Could you check a few things on this model? Use its own coordinates, in mm. Face numbers are marked on the shaded views. A direction names the side the tool comes from. Round coordinates to 2 decimals unless told otherwise and drop trailing zeros. Write each loop counter-clockwise with the first axis right and the second up, starting at its lowest first coordinate (ties: lowest second). Pieces come first, ordered by that corner, then holes. Notation, with made-up numbers: (52.25, 0.25) -> (67.25, 0.25) arc R33 cw to (67.25, 30.25) -> close; hole circle Ø8 at (71, -1.75). An arc over 180 degrees is marked (long way). Answer in a Markdown table with one row per item.
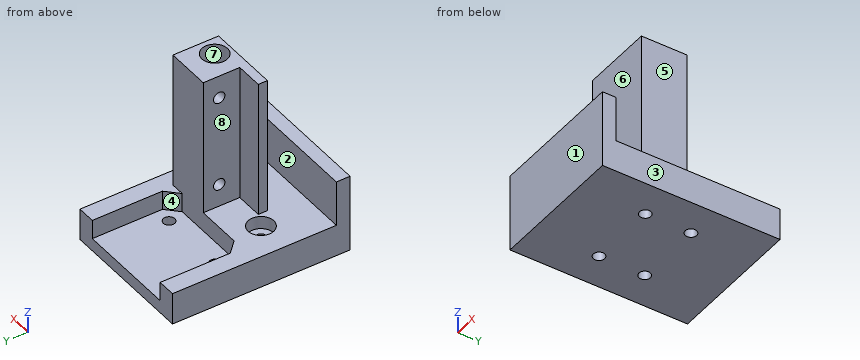
from build123d import *

# Parameters (mm, degrees)
SKETCH016_W     = 30
SKETCH016_H     = 38.9
SKETCH016_R     = 1.25
PAD010_DEPTH    = 7
POCKET005_DEPTH = 4.2
SKETCH020_R     = 2.8
POCKET006_DEPTH = 2.8
SKETCH021_R     = 2.8
PAD011_DEPTH    = 30
SKETCH022_R     = 1.25
POCKET007_DEPTH = 5.3
SKETCH026_W     = 30
SKETCH026_H     = 3
PAD015_DEPTH    = 10


with BuildPart() as part:
    # Sketch016 (on Face1 of ReferencePad007) → Pad010 (new body)
    with BuildSketch(Plane.XY.offset(3.5)):
        with Locations((0, 132.225)):
            Rectangle(SKETCH016_W, SKETCH016_H)
        with Locations((-7.5, 137.225)):
            Circle(SKETCH016_R, mode=Mode.SUBTRACT)
        with Locations((-7.5, 127.225)):
            Circle(SKETCH016_R, mode=Mode.SUBTRACT)
        with Locations((7.5, 137.225)):
            Circle(SKETCH016_R, mode=Mode.SUBTRACT)
        with Locations((7.5, 127.225)):
            Circle(SKETCH016_R, mode=Mode.SUBTRACT)
    extrude(amount=PAD010_DEPTH)

    # Sketch019 (on Face10 of Pad010) → Pocket005 (cut)
    with BuildSketch(Plane.XY.offset(10.5)):
        Polygon((-8.411624, 133.725), (-11, 136.313376), (-11, 151.675), (11, 151.675), (11, 136.313376), (8.411624, 133.725), align=None)
    extrude(amount=-POCKET005_DEPTH, mode=Mode.SUBTRACT)

    # Sketch020 (on Face5 of Pocket005) → Pocket006 (cut)
    with BuildSketch(Plane.XY.offset(10.5)):
        with Locations((-7.5, 127.225)):
            Circle(SKETCH020_R)
        with Locations((7.5, 127.225)):
            Circle(SKETCH020_R)
    extrude(amount=-POCKET006_DEPTH, mode=Mode.SUBTRACT)

    # Sketch021 (on Face5 of Pocket006) → Pad011 (join)
    with BuildSketch(Plane.XY.offset(10.5)):
        Polygon((-4.411624, 123.725), (11.411624, 123.725), (11.411624, 133.725), (1.588376, 133.725), (1.588376, 125.725), (-4.411624, 125.725), align=None)
        with Locations((7.5, 127.225)):
            Circle(SKETCH021_R, mode=Mode.SUBTRACT)
    extrude(amount=PAD011_DEPTH)

    # Sketch022 (on Face14 of Pad011) → Pocket007 (cut)
    with BuildSketch(Plane(origin=(1.588376, 0, 8), x_dir=(0, -1, 0), z_dir=(-1, 0, 0))):
        with Locations((-130.225, 27.5)):
            Circle(SKETCH022_R)
        with Locations((-130.225, 7.5)):
            Circle(SKETCH022_R)
    extrude(amount=-POCKET007_DEPTH, mode=Mode.SUBTRACT)

    # Sketch026 (on Face5 of Pocket007) → Pad015 (join)
    with BuildSketch(Plane.XY.offset(10.5)):
        with Locations((0, 114.275)):
            Rectangle(SKETCH026_W, SKETCH026_H)
    extrude(amount=PAD015_DEPTH)


solid = part.part
1) Thinking about a two-plate mould opening in Y: for the marked faces 1, 2 and 3, which applies, +Y half, -Y half, draft (parallel to the pull), parting line (faces both ways), or undercut?
Findings:
| item | result |
|---|---|
| face 1 | -Y half |
| face 2 | undercut |
| face 3 | draft |
2) Please list where these lines run through material, in increasing order: line 1 (Y direction, x = 7.5, z = 5.65) (3 decimals); line 2 (Y direction, x = 7.5, z = 26) (3 decimals); line 3 (Y direction, x = 3.9, z = 35.5) (3 decimals).
Findings:
| item | result |
|---|---|
| line 1 | y = 112.775 to 125.975, 128.475 to 135.975, 138.475 to 151.675 |
| line 2 | y = 123.725 to 124.425, 130.025 to 133.725 |
| line 3 | y = 123.725 to 128.975, 131.475 to 133.725 |
3) Imagine slicing it at B-B, the plane z = 12. Please give me the cut outline in (x, y) (3 decimals).
Findings:
| item | result |
|---|---|
| outline | (-15, 112.775) -> (15, 112.775) -> (15, 115.775) -> (-15, 115.775) -> close; (-4.412, 123.725) -> (11.412, 123.725) -> (11.412, 133.725) -> (1.588, 133.725) -> (1.588, 125.725) -> (-4.412, 125.725) -> close; hole circle Ø5.6 at (7.5, 127.225) |
4) For the marked faces 4, 5, 6, 7 and 8, which set-ups out of +Z, -Z, +X, -X, +Y, -Y let a thin tool reach every point of the face, with its end or its side?
Findings:
| item | result |
|---|---|
| face 4 | +Z, +Y |
| face 5 | +Z, +X, +Y |
| face 6 | +Z, +X, -X |
| face 7 | +Z |
| face 8 | +Z, -X, +Y |
5) Imagine slicing it at A-A, the plane x = 7.5. Please give me the cut outline in (y, z) (3 decimals), plus the area to 3 significant figures.
Findings:
| item | result |
|---|---|
| outline | (112.775, 3.5) -> (125.975, 3.5) -> (125.975, 7.7) -> (124.425, 7.7) -> (124.425, 40.5) -> (123.725, 40.5) -> (123.725, 10.5) -> (115.775, 10.5) -> (115.775, 20.5) -> (112.775, 20.5) -> close; (128.475, 3.5) -> (135.975, 3.5) -> (135.975, 6.3) -> (133.725, 6.3) -> (133.725, 40.5) -> (130.025, 40.5) -> (130.025, 7.7) -> (128.475, 7.7) -> close; (138.475, 3.5) -> (151.675, 3.5) -> (151.675, 6.3) -> (138.475, 6.3) -> close |
| area | 326 mm^2 |
6) Imagine slicing it at C-C, the plane x = -0.5. Please give me the cut outline in (y, z) (3 decimals).
Findings:
| item | result |
|---|---|
| outline | (112.775, 3.5) -> (151.675, 3.5) -> (151.675, 6.3) -> (133.725, 6.3) -> (133.725, 10.5) -> (125.725, 10.5) -> (125.725, 40.5) -> (123.725, 40.5) -> (123.725, 10.5) -> (115.775, 10.5) -> (115.775, 20.5) -> (112.775, 20.5) -> close |
7) Imagine slicing it at D-D, the plane z = 28.5. Please give me the cut outline in (x, y) (3 decimals), plus the area to 3 significant figures.
Findings:
| item | result |
|---|---|
| outline | (-4.412, 123.725) -> (11.412, 123.725) -> (11.412, 133.725) -> (1.588, 133.725) -> (1.588, 125.725) -> (-4.412, 125.725) -> close; hole circle Ø5.6 at (7.5, 127.225) |
| area | 85.6 mm^2 |
8) For pin 1 (3 mm diameter, centred on x = -0.5, z = 14.5, fed in from +Y) (3 decimals); pin 2 (4 mm diameter, centred on y = 130.225, z = 15.5, fed in from +X); pin 3 (2 mm diameter, centred on x = -2.5, z = 7.5, fed in from +Y) (3 decimals), each with a flat end and sliding along its axis, tell me the tip position at first contact or that it passes through.
Findings:
| item | result |
|---|---|
| pin 1 | stops at y = 125.725 |
| pin 2 | stops at x = 11.41 |
| pin 3 | stops at y = 133.725 |
